For this review, take the finished solid that the model builds, in its own axes (mm). Face numbers are marked on the shaded views. A direction names the side the tool comes from. Give positions to 0.01 mm unless a question says otherwise; leave off trailing zeros. Write each loop counter-clockwise with the first axis right and the second up, starting at its lowest first coordinate (ties: lowest second). Pieces come first, ordered by that corner, then holes.
1) Machinability: for the marked faces 1, 2 and 3, which of the approach directions +Z, -Z, +X, -X, +Y, -Y give a long, thin tool a straight path to every point of the face, cutting with its end or side? Answer none if there is none.
2) For P1, Ø1.5, axis at y = 7.5, z = 2, coming from the -X side; P2, Ø8, axis at y = 8.5, z = 2, coming from the -X side; P3, Ø9, axis at x = -6, y = 3, coming from the -Z side, all flat-tipped, find the tip position at first contact; note any pin that passes through.
3) Draft analysis for pull direction Y (two halves, no side actions). For the marked faces 4, 5 and 6, state which applies: pulls with the +Y half, pulls with the -Y half, needs draft (parallel to the pull), parting line crosses it, or undercut.
4) Wall thickness on line 1 along Y through (x, z) = (5.5, 4); line 2 along Y through (x, z) = (2.5, 1.75); line 3 along Y through (x, z) = (17, -7.5): over which ranges is each line inside the solid? List them lowest first.
5) We need section A-A on y = 11. Give the boundary of the cut face in (x, z), and give its area (3 significant figures).
6) We need section D-D on y = -6. Give the boundary of the cut face in (x, z).
7) We need section C-C on z = -13.5. Give the boundary of the cut face in (x, y), and give its area (3 significant figures).
8) We need section B-B on x = 3. Give the boundary of the cut face in (y, z).
from build123d import *

# Parameters (mm, degrees)
ESQUISSE1_W             = 40
ESQUISSE1_H             = 30
BOSS_EXTRU_1_DEPTH      = 5
ESQUISSE4_W             = 40
ESQUISSE4_H             = 25
BOSS_EXTRU_2_DEPTH      = 4
ESQUISSE5_W             = 23
ESQUISSE5_H             = 12
ENL_V_MAT_EXTRU_2_DEPTH = 5
ESQUISSE6_R             = 10
ENL_V_MAT_EXTRU_3_DEPTH = 2
ENL_V_START             = -34
ENL_V_MAT_EXTRU_4_DEPTH = 34


# Read off the part's stored shape, not the designer's step: Enlèv. mat.-Extru.4
with BuildPart() as part:
    # Esquisse1 → Boss.-Extru.1 (new body)
    with BuildSketch(Plane.XY):
        Rectangle(ESQUISSE1_W, ESQUISSE1_H)
    extrude(amount=BOSS_EXTRU_1_DEPTH)

    # Esquisse4 → Boss.-Extru.2 (add)
    with BuildSketch(Plane.XZ.offset(15)):
        with Locations((0, -7.5)):
            Rectangle(ESQUISSE4_W, ESQUISSE4_H)
    extrude(amount=BOSS_EXTRU_2_DEPTH)

    # Esquisse5 → Enlèv. mat.-Extru.2 (cut)
    with BuildSketch(Plane(origin=(0, 0, 0), x_dir=(-1, 0, 0), z_dir=(0, 0, -1))):
        with Locations((0, 7)):
            Rectangle(ESQUISSE5_W, ESQUISSE5_H)
    extrude(amount=-ENL_V_MAT_EXTRU_2_DEPTH, mode=Mode.SUBTRACT)

    # Esquisse6 → Enlèv. mat.-Extru.3 (cut)
    with BuildSketch(Plane.XZ.offset(19)):
        with Locations(Location((-0.043131573, -7.485697827, 0), (0, 0, 270))):
            Circle(ESQUISSE6_R)
    extrude(amount=-ENL_V_MAT_EXTRU_3_DEPTH, mode=Mode.SUBTRACT)

    # Enlèv. mat.-Extru.4 outline → Enlèv. mat.-Extru.4 (cut)
    with BuildSketch(Plane.XZ.offset(19).offset(ENL_V_START)):
        with BuildLine():
            ThreePointArc((14.935431434, 5), (19.456859524, -7.504332113), (14.911541313, -20))
            Line((14.911541313, -20), (20, -20))
            Line((20, -20), (20, 5))
            Line((20, 5), (14.935431434, 5))
        make_face()
        with BuildLine():
            Line((-20, -20), (-14.997804459, -20))
            ThreePointArc((-14.997804459, -20), (-19.543122669, -7.504332113), (-15.02169458, 5))
            Line((-15.02169458, 5), (-20, 5))
            Line((-20, 5), (-20, -20))
        make_face()
    extrude(amount=ENL_V_MAT_EXTRU_4_DEPTH, mode=Mode.SUBTRACT)


solid = part.part
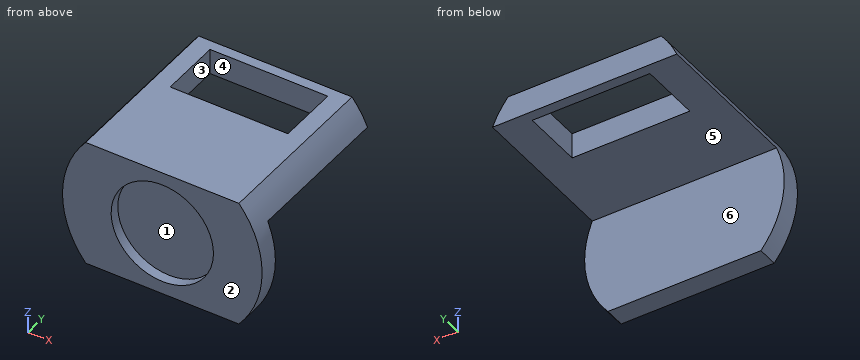
Results list:
1. face 1: -Y
1. face 2: +Z, -Z, +X, -X, -Y
1. face 3: +Z, -Z
2. P1: stops at x = -17.48
2. P2: stops at x = -18.05
2. P3: stops at z = 0
3. face 4: undercut
3. face 5: needs draft
3. face 6: pulls with the +Y half
4. line 1: y = -19 to 1, 13 to 15
4. line 2: y = -17 to 1, 13 to 15
4. line 3: y = -19 to -15
5. outline: (-18.05, 0) - (-11.5, 0) - (-11.5, 5) - (-15.02, 5) arc R19.5 ccw to start; (11.5, 0) - (17.96, 0) arc R19.5 ccw to (14.94, 5) - (11.5, 5) - close
5. area: 51.6 mm2
6. outline: (-18.05, 0) - (17.96, 0) arc R19.5 ccw to (14.94, 5) - (-15.02, 5) arc R19.5 ccw to start
7. outline: (-18.59, -19) - (-8.03, -19) - (-8.03, -17) - (7.95, -17) - (7.95, -19) - (18.51, -19) - (18.51, -15) - (-18.59, -15) - close
7. area: 116 mm2
8. outline: (-19, -20) - (-15, -20) - (-15, 0) - (1, 0) - (1, 5) - (-19, 5) - (-19, 2.04) - (-17, 2.04) - (-17, -17.01) - (-19, -17.01) - close; (13, 0) - (15, 0) - (15, 5) - (13, 5) - close
